from build123d import *

# Parameters (mm, degrees)
F1_DEPTH = 2


with BuildPart() as f1:
    # F0 (on Top) → F1 (new body)
    with BuildSketch(Plane.XY):
        with BuildLine():
            Line((35, 0), (5, 0))
            ThreePointArc((5, 0), (0, -5), (-5, 0))
            Line((-5, 0), (-35, 0))
            ThreePointArc((-35, 0), (0, -35), (35, 0))
        make_face()
        with BuildLine():
            Line((47, 0), (35, 0))
            ThreePointArc((35, 0), (0, -35), (-35, 0))
            Line((-35, 0), (-40, 0))
            Line((-40, 0), (-40, -37.5692024827))
            Line((-40, -37.5692024827), (47, -37.5692024827))
            Line((47, -37.5692024827), (47, 0))
        make_face()
    extrude(amount=F1_DEPTH)


solid = f1.part
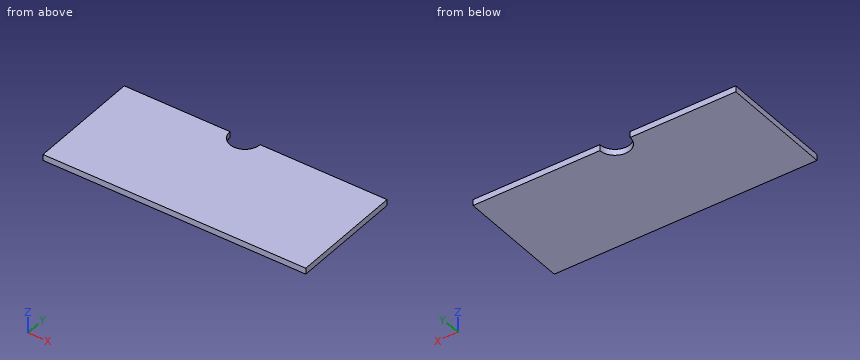
Geometry check sheet. Reference: the model listing, model coordinates, mm. Give positions to 0.01 mm unless a question says otherwise; leave off trailing zeros. Write each loop counter-clockwise with the first axis right and the second up, starting at its lowest first coordinate (ties: lowest second). Pieces come first, ordered by that corner, then holes.
1) Go/stop test with a flat-tipped pin: pin 1 Ø5 at (x, y) = (-5.5, -22) entering from -Z. Record where the tip stops, or that it passes through.
Values follow:
pin 1: stops at z = 0
2) Cross-section at B-B (x = 0). Record the boundary of the cut face in (y, z), plus the area to 3 significant figures.
Values follow:
outline: (-37.57, 0) - (-5, 0) - (-5, 2) - (-37.57, 2) - close
area: 65.1 mm2
3) Cross-section at A-A (y = -3.5). Record the boundary of the cut face in (x, z), plus the area to 3 significant figures.
Values follow:
outline: (-40, 0) - (-3.57, 0) - (-3.57, 2) - (-40, 2) - close; (3.57, 0) - (47, 0) - (47, 2) - (3.57, 2) - close
area: 160 mm2
4) Thickness scan on line 1 (X direction, y = -3, z = 0.85); line 2 (X direction, y = -4.5, z = 1.5); line 3 (Y direction, x = -3, z = 0.8). Record the ranges inside material, lowest first.
Values follow:
line 1: x = -40 to -4, 4 to 47
line 2: x = -40 to -2.18, 2.18 to 47
line 3: y = -37.57 to -4
